Source: CAD feature listing. Evaluate the final solid. Frame: model axes, mm. A direction names the side the tool comes from. Give positions to 0.01 mm unless a question says otherwise; leave off trailing zeros. Loops run counter-clockwise (first coordinate to the right, second up) from the corner with the lowest first, then second, coordinate; pieces in that order, holes last. Notation, with made-up numbers: M -22,43 L 3,43 A35 cw 3,81 Z; hole C 64.25,-38 d3. An arc over 180 degrees is marked long. Answer in a Markdown table with one row per item.
```python
from build123d import *

# Parameters (mm, degrees)
F0_R     = 2
F0_R_2   = 7.5
F1_DEPTH = 10
F3_DEPTH = 169
F4_W     = 223
F4_H     = 143
F4_W_2   = 212.9999995232
F4_H_2   = 132.9999995232
F5_DEPTH = 5
F6_DEPTH = 25
F7_R     = 4.5
F8_DEPTH = 25


with BuildPart() as f1:
    # F0 (on Top) → F1 (new body)
    with BuildSketch(Plane.XY):
        with BuildLine():
            Line((129.5, 134.5), (-129.5, 134.5))
            ThreePointArc((-129.5, 134.5), (-133.0355339059, 133.0355339059), (-134.5, 129.5))
            Line((-134.5, 129.5), (-134.5, -129.5))
            ThreePointArc((-134.5, -129.5), (-133.0355339059, -133.0355339059), (-129.5, -134.5))
            Line((-129.5, -134.5), (129.5, -134.5))
            ThreePointArc((129.5, -134.5), (133.0355339059, -133.0355339059), (134.5, -129.5))
            Line((134.5, -129.5), (134.5, 129.5))
            ThreePointArc((134.5, 129.5), (133.0355339059, 133.0355339059), (129.5, 134.5))
        make_face()
        with Locations((-12.124355653, -7)):
            Circle(F0_R, mode=Mode.SUBTRACT)
        with Locations((0, -14)):
            Circle(F0_R, mode=Mode.SUBTRACT)
        with Locations((12.124355653, -7)):
            Circle(F0_R, mode=Mode.SUBTRACT)
        with Locations((-12.124355653, 7)):
            Circle(F0_R, mode=Mode.SUBTRACT)
        Circle(F0_R_2, mode=Mode.SUBTRACT)
        with Locations((12.124355653, 7)):
            Circle(F0_R, mode=Mode.SUBTRACT)
        with Locations((0, 14)):
            Circle(F0_R, mode=Mode.SUBTRACT)
    extrude(amount=F1_DEPTH)

    # F2 (on face) → F3 (join)
    with BuildSketch(Plane.XY.offset(10)):
        with BuildLine():
            ThreePointArc((-134.5, -129.5), (-133.0355339059, -133.0355339059), (-129.5, -134.5))
            Line((-129.5, -134.5), (129.5, -134.5))
            ThreePointArc((129.5, -134.5), (133.0355339059, -133.0355339059), (134.5, -129.5))
            Line((134.5, -129.5), (134.5, -119.5))
            Line((134.5, -119.5), (134.5, 129.5))
            ThreePointArc((134.5, 129.5), (133.0355339059, 133.0355339059), (129.5, 134.5))
            Line((129.5, 134.5), (119.5, 134.5))
            Line((119.5, 134.5), (119.5, -119.5))
            Line((119.5, -119.5), (-119.5, -119.5))
            Line((-119.5, -119.5), (-119.5, 134.5))
            Line((-119.5, 134.5), (-129.5, 134.5))
            ThreePointArc((-129.5, 134.5), (-133.0355339059, 133.0355339059), (-134.5, 129.5))
            Line((-134.5, 129.5), (-134.5, -119.5))
            Line((-134.5, -119.5), (-134.5, -129.5))
        make_face()
    extrude(amount=F3_DEPTH)

    # F4 (on face) → F5 (cut)
    with BuildSketch(Plane.XZ.offset(134.5)):
        with Locations((0, 89.5)):
            Rectangle(F4_W, F4_H)
        with Locations((0, 89.5)):
            Rectangle(F4_W_2, F4_H_2, mode=Mode.SUBTRACT)
    extrude(amount=-F5_DEPTH, mode=Mode.SUBTRACT)

    # F6 (cut): a face of the model
    f6_faces = [f1.faces().sort_by_distance(p)[0] for p in [
        (0, -134.5, 89.5),
    ]]
    extrude(f6_faces, amount=-F6_DEPTH, mode=Mode.SUBTRACT)

    # F7 (on face) → F8 (cut)
    with BuildSketch(Plane(origin=(0, -119.5, 0), x_dir=(-1, 0, 0), z_dir=(0, 1, 0))):
        with Locations((-45, 169.7952974686)):
            Circle(F7_R)
        with Locations((45, 169.7952974686)):
            Circle(F7_R)
    extrude(amount=-F8_DEPTH, mode=Mode.SUBTRACT)


solid = f1.part
```
1) Set-up query: faces 1 (the flat face through (106.5, -125, 89)), 2 (the flat face through (-9, -129.5, 21)), 3 (the flat face through (-2, 9, 10)). Return all of +Z, -Z, +X, -X, +Y, -Y with unobstructed straight access to the full face (end or side cutting, diameter ignored); none if empty.
Reply:
| item | result |
|---|---|
| face 1 | +Y, -Y |
| face 2 | -Y |
| face 3 | +Z, +Y |
2) Section C-C, the plane x = -45. Return loops of the section in (y, z).
Reply:
| item | result |
|---|---|
| outline | M -134.5,0 L 134.5,0 L 134.5,10 L -119.5,10 L -119.5,23 L -129.5,23 L -129.5,18 L -134.5,18 Z; M -134.5,161 L -129.5,161 L -129.5,156 L -119.5,156 L -119.5,165.3 L -134.5,165.3 Z; M -134.5,174.3 L -119.5,174.3 L -119.5,179 L -134.5,179 Z |
3) Pull-direction query (X, two-part tool) for faces 4 (the flat face through (-2, -134.5, 168)), 5 (the flat face through (-134.5, 2, 88)), 6 (the flat face through (119.5, 9, 93)); classes: released by +X, released by -X, zero draft, split by the parting line, or undercut.
Reply:
| item | result |
|---|---|
| face 4 | zero draft |
| face 5 | released by -X |
| face 6 | undercut |
4) Section A-A, the plane z = 84. Return loops of the section in (x, y).
Reply:
| item | result |
|---|---|
| outline | M -134.5,-129.5 A5 ccw -129.5,-134.5 L -111.5,-134.5 L -111.5,-129.5 L -106.5,-129.5 L -106.5,-119.5 L -119.5,-119.5 L -119.5,134.5 L -129.5,134.5 A5 ccw -134.5,129.5 Z; M 106.5,-129.5 L 111.5,-129.5 L 111.5,-134.5 L 129.5,-134.5 A5 ccw 134.5,-129.5 L 134.5,129.5 A5 ccw 129.5,134.5 L 119.5,134.5 L 119.5,-119.5 L 106.5,-119.5 Z |
5) Section B-B, the plane y = 0. Return loops of the section in (x, z), then the cut area to 3 significant figures.
Reply:
| item | result |
|---|---|
| outline | M -134.5,0 L -7.5,0 L -7.5,10 L -119.5,10 L -119.5,179 L -134.5,179 Z; M 7.5,0 L 134.5,0 L 134.5,179 L 119.5,179 L 119.5,10 L 7.5,10 Z |
| area | 7,610 mm² |
6) Pin query (flat end, axial travel): pin 1 Ø6.5 at (x, y) = (-12.12, -7) entering from +Z; pin 2 Ø2.5 at (x, y) = (12.12, -7) entering from -Z. Return the tip coordinate at first contact, or that it passes through.
Reply:
| item | result |
|---|---|
| pin 1 | stops at z = 10 |
| pin 2 | passes through |
7) Section D-D, the plane x = 74.5. Return loops of the section in (y, z), then the cut area to 3 significant figures.
Reply:
| item | result |
|---|---|
| outline | M -134.5,0 L 134.5,0 L 134.5,10 L -119.5,10 L -119.5,23 L -129.5,23 L -129.5,18 L -134.5,18 Z; M -134.5,161 L -129.5,161 L -129.5,156 L -119.5,156 L -119.5,179 L -134.5,179 Z |
| area | 3,180 mm² |
8) Material intervals for L1, parallel to Z at x = -45, y = -130; L2, parallel to Y at x = 0, z = 4.5; L3, parallel to Z at x = 45, y = -126, sorted ascending.
Reply:
| item | result |
|---|---|
| L1 | z = 0 to 18, 161 to 165.3, 174.3 to 179 |
| L2 | y = -134.5 to -16, -12 to -7.5, 7.5 to 12, 16 to 134.5 |
| L3 | z = 0 to 23, 156 to 165.3, 174.3 to 179 |
